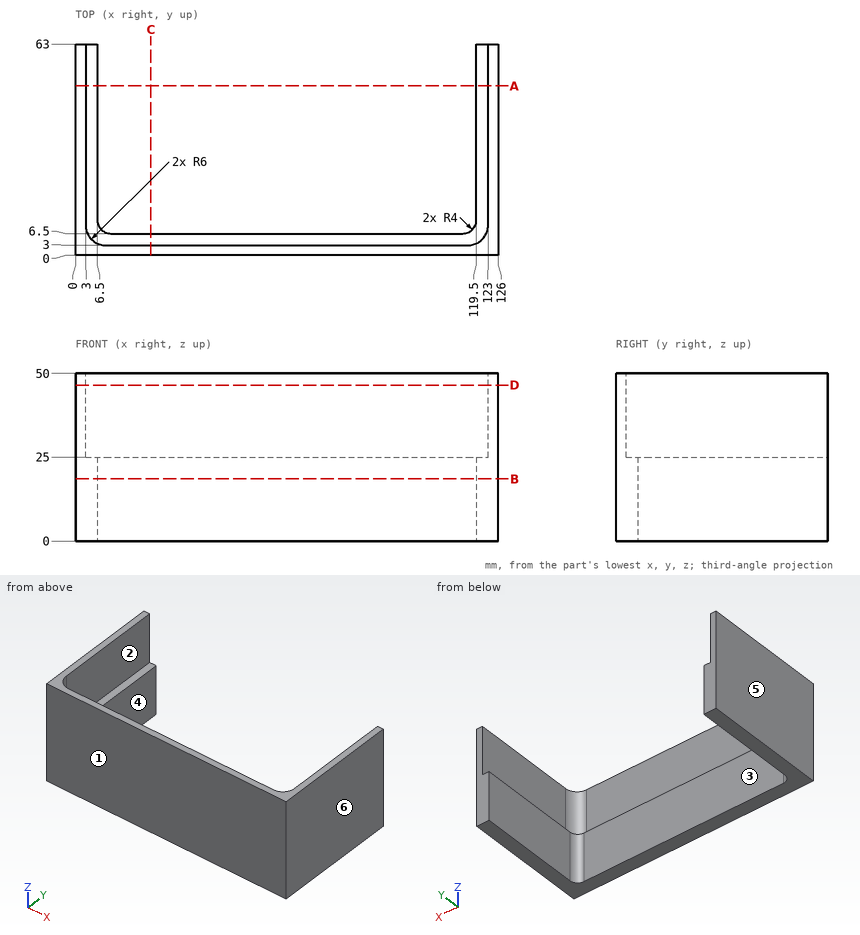
Check sheet for the drawn part. Datum: minimum x, y, z corner. Units: mm. A direction names the side the tool comes from. Coordinates: 2 decimals unless noted, no trailing zeros. Loops run counter-clockwise (first coordinate to the right, second up) from the corner with the lowest first, then second, coordinate; pieces in that order, holes last. Notation, with made-up numbers: (61.25, -15.75) -> (92.25, -15.75) arc R21 ccw to (92.25, -6.75) -> close; hole circle Ø4 at (28, 37.5). An arc over 180 degrees is marked (long way). Answer in a Markdown table with one row per item.
1) Scan lines: line 1 along X through (y, z) = (28, 38); line 2 along X through (y, z) = (48, 4.5); line 3 along Y through (x, z) = (65.5, 32.5). Record each from-to range of solid material in increasing order. Write a range as from..to.
The answers:
| item | result |
|---|---|
| line 1 | x = 0..3, 123..126 |
| line 2 | x = 0..6.5, 119.5..126 |
| line 3 | y = 0..3 |
2) Access from +Z, -Z, +X, -X, +Y, -Y to the whole of each face (thin tool, end or side, straight path). Record for the marked faces 1, 2 and 3.
The answers:
| item | result |
|---|---|
| face 1 | +Z, -Z, +X, -X, -Y |
| face 2 | +Z, +Y |
| face 3 | +Z, -Z, +Y |
3) Draft check along X on the marked faces 4, 5 and 6. Enter one of: released by +X, released by -X, zero draft, split by the parting line, or undercut.
The answers:
| item | result |
|---|---|
| face 4 | undercut |
| face 5 | released by -X |
| face 6 | released by +X |
4) Section check C-C (x = 22.5). Record the cut outline in (y, z).
The answers:
| item | result |
|---|---|
| outline | (0, 0) -> (6.5, 0) -> (6.5, 25) -> (3, 25) -> (3, 50) -> (0, 50) -> close |
5) Section check A-A (y = 50.5). Record the cut outline in (x, z).
The answers:
| item | result |
|---|---|
| outline | (0, 0) -> (6.5, 0) -> (6.5, 25) -> (3, 25) -> (3, 50) -> (0, 50) -> close; (119.5, 0) -> (126, 0) -> (126, 50) -> (123, 50) -> (123, 25) -> (119.5, 25) -> close |
6) Depth check by flat-ended pin: P1, Ø2, axis at x = 54, z = 14, coming from the -Y side; P2, Ø1, axis at x = 101, z = 16.5, coming from the +Y side; P3, Ø3, axis at x = 28.5, y = 8.5, coming from the +Z side; P4, Ø12.5, axis at x = 80, z = 43.5, coming from the +Y side. Enter the tip coordinate at first touch or a pass-through.
The answers:
| item | result |
|---|---|
| P1 | stops at y = 0 |
| P2 | stops at y = 6.5 |
| P3 | passes through |
| P4 | stops at y = 3 |
7) Section check B-B (z = 18.5). Record the cut outline in (x, y), and give its area (3 significant figures).
The answers:
| item | result |
|---|---|
| outline | (0, 0) -> (126, 0) -> (126, 63) -> (119.5, 63) -> (119.5, 10.5) arc R4 cw to (115.5, 6.5) -> (10.5, 6.5) arc R4 cw to (6.5, 10.5) -> (6.5, 63) -> (0, 63) -> close |
| area | 1,560 mm2 |
8) Section check D-D (z = 46.5). Record the cut outline in (x, y), and give its area (3 significant figures).
The answers:
| item | result |
|---|---|
| outline | (0, 0) -> (126, 0) -> (126, 63) -> (123, 63) -> (123, 9) arc R6 cw to (117, 3) -> (9, 3) arc R6 cw to (3, 9) -> (3, 63) -> (0, 63) -> close |
| area | 753 mm2 |
